from build123d import *

# Parameters (mm, degrees)
SKETCH1_R                = 1.4
BOSS_EXTRUDE1_DEPTH      = 24
SKETCH2_R                = 2.5
BOSS_EXTRUDE2_DEPTH      = 60
SKETCH3_R                = 1.4
BOSS_EXTRUDE3_DEPTH      = 24
SKETCH4_W                = 15
SKETCH4_H                = 30
BOSS_EXTRUDE4_DEPTH      = 1.5
BOSS_EXTRUDE4_DEPTH_BACK = 1.5
SKETCH5_W                = 10
SKETCH5_H                = 10
CUT_EXTRUDE1_DEPTH       = 10
CUT_EXTRUDE1_DEPTH_BACK  = 7


with BuildPart() as part:
    # Sketch1 → Boss-Extrude1 (new body)
    with BuildSketch(Plane(origin=(0, 0, 0), x_dir=(0, 0, -1), z_dir=(1, 0, 0))):
        Circle(SKETCH1_R)
    extrude(amount=BOSS_EXTRUDE1_DEPTH)

    # Sketch2 → Boss-Extrude2 (add)
    with BuildSketch(Plane(origin=(24, 0, 0), x_dir=(0, 0, -1), z_dir=(1, 0, 0))):
        Circle(SKETCH2_R)
    extrude(amount=BOSS_EXTRUDE2_DEPTH)

    # Sketch3 → Boss-Extrude3 (add)
    with BuildSketch(Plane(origin=(84, 0, 0), x_dir=(0, 0, -1), z_dir=(1, 0, 0))):
        Circle(SKETCH3_R)
    extrude(amount=BOSS_EXTRUDE3_DEPTH)

    # Sketch4 → Boss-Extrude4 (add, two sides)
    with BuildSketch(Plane.XY) as boss_extrude4_sk:
        with Locations((74.346083047, -16.435117581)):
            Rectangle(SKETCH4_W, SKETCH4_H)
    extrude(amount=BOSS_EXTRUDE4_DEPTH)
    extrude(boss_extrude4_sk.sketch, amount=-BOSS_EXTRUDE4_DEPTH_BACK)

    # Sketch5 → Cut-Extrude1 (cut, two sides)
    with BuildSketch(Plane(origin=(0, 0, -1.5), x_dir=(-1, 0, 0), z_dir=(0, 0, -1))) as cut_extrude1_sk:
        with Locations((-74.346083047, -14.5)):
            Rectangle(SKETCH5_W, SKETCH5_H)
        with BuildLine():
            Line((-79.346083047, -25.5), (-69.346083047, -25.5))
            ThreePointArc((-69.346083047, -25.5), (-67.696083047, -27.15), (-69.346083047, -28.8))
            Line((-69.346083047, -28.8), (-79.346083047, -28.8))
            ThreePointArc((-79.346083047, -28.8), (-80.996083047, -27.15), (-79.346083047, -25.5))
        make_face()
    extrude(amount=CUT_EXTRUDE1_DEPTH, mode=Mode.SUBTRACT)
    extrude(cut_extrude1_sk.sketch, amount=-CUT_EXTRUDE1_DEPTH_BACK, mode=Mode.SUBTRACT)


solid = part.part
The listing builds one solid part. Answer for the finished solid, in the listing's coordinates (mm). A direction names the side the tool comes from. Round coordinates to 2 decimals unless told otherwise and drop trailing zeros. Order: outer loops, then holes, each group sorted by start corner. A loop starts at its lowest first (then second) coordinate and runs counter-clockwise, first axis right, second up. Notation, with made-up numbers: (-27, 76) -> (17, 76) arc R28 ccw to (17, 94) -> close; hole circle Ø6 at (-38.75, 64.5). An arc over 180 degrees is marked (long way). Write each question's results on one line, items separated by ' | '. Start each with the question number.
Q1. Find section C-C (y = 0). Determine the outline of the cut face in (x, z), then the cut area to 3 significant figures.
Q2. Straight lines are drawn through the part: probe 1 along X at (y, z) = (-16.5, 1.2); probe 2 along X at (y, z) = (-20.5, 0.15); probe 3 along X at (y, z) = (0, -2). For each, find the intervals that lie inside material, in ascending order. Write a range as from..to.
Q3. Find section A-A (y = -15.5). Determine the outline of the cut face in (x, z).
Q4. Which of the six approach directions +Z, -Z, +X, -X, +Y, -Y give full straight-line access (tool end or side, diameter ignored) to faces 5 (the cylindrical face through (11.83, 0.06, 1.4)), 6 (the flat face through (84, -1.1, -1.1)), 7 (the flat face through (74, -9.5, 0))?
Q5. Find section B-B (z = 0). Determine the outline of the cut face in (x, y), then the cut area to 3 significant figures.
Q6. Find section D-D (x = 9). Determine the outline of the cut face in (y, z).
Q7. The mould has two halves that part along X. Classify faces 1 (the cylindrical face through (80.996, -27.186, -0.021)), 2 (the flat face through (74, -25.5, 0)), 3 (the flat face through (81.846, -17, 0)), 4 (the flat face through (66.846, -17, 0)): pulls with the +X half, pulls with the -X half, needs draft (parallel to the pull), parting line crosses it, or undercut.
Q8. Each of these flat-tipped pins is pushed along its axis until it touches: pin 1 (12 mm diameter, centred on x = 76.5, y = -10.5, fed in from -Z); pin 2 (2 mm diameter, centred on x = 80, y = -19.5, fed in from +Z); pin 3 (2.5 mm diameter, centred on y = -24, z = 0, fed in from +X). Where does it stop, or does it pass through?
Worked answers:
1) outline: (0, -1.4) -> (24, -1.4) -> (24, -2.5) -> (84, -2.5) -> (84, -1.4) -> (108, -1.4) -> (108, 1.4) -> (84, 1.4) -> (84, 2.5) -> (24, 2.5) -> (24, 1.4) -> (0, 1.4) -> close | area: 434 mm2
2) probe 1: x = 66.85..69.35, 79.35..81.85 | probe 2: x = 66.85..81.85 | probe 3: x = 24..84
3) outline: (66.85, -1.5) -> (69.35, -1.5) -> (69.35, 1.5) -> (66.85, 1.5) -> close; (79.35, -1.5) -> (81.85, -1.5) -> (81.85, 1.5) -> (79.35, 1.5) -> close
4) face 5: -X | face 6: +X | face 7: +Z, -Z
5) outline: (0, -1.4) -> (24, -1.4) -> (24, -2.5) -> (66.85, -2.5) -> (66.85, -31.44) -> (81.85, -31.44) -> (81.85, -2.5) -> (84, -2.5) -> (84, -1.4) -> (108, -1.4) -> (108, 1.4) -> (84, 1.4) -> (84, 2.5) -> (24, 2.5) -> (24, 1.4) -> (0, 1.4) -> close; hole (69.35, -28.8) -> (79.35, -28.8) arc R1.65 ccw to (79.35, -25.5) -> (69.35, -25.5) arc R1.65 ccw to start; hole (69.35, -19.5) -> (79.35, -19.5) -> (79.35, -9.5) -> (69.35, -9.5) -> close | area: 727 mm2
6) outline: circle Ø2.8 at (0, 0)
7) face 1: undercut | face 2: undercut | face 3: pulls with the +X half | face 4: pulls with the -X half
8) pin 1: stops at z = -1.5 | pin 2: stops at z = 1.5 | pin 3: stops at x = 81.85
